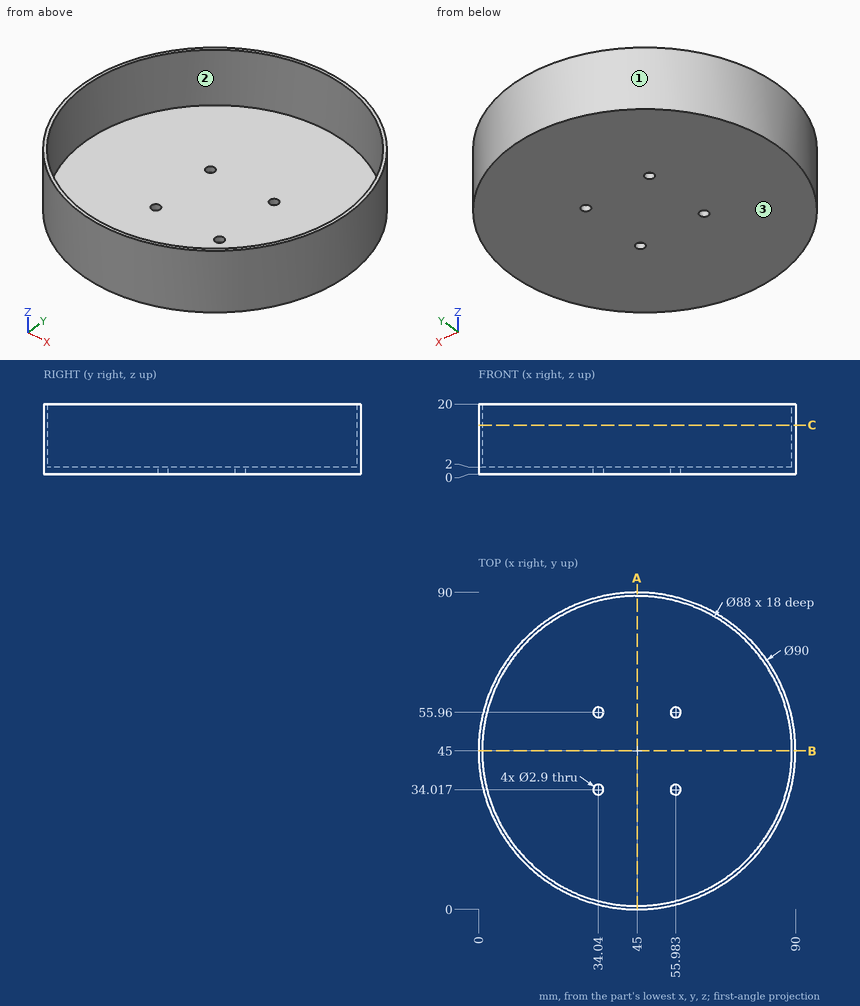
Study the drawing (mm; zero at the part's minimum x, y, z) and answer. Coordinates: 2 decimals unless noted, no trailing zeros. Order: outer loops, then holes, each group sorted by start corner. A loop starts at its lowest first (then second) coordinate and runs counter-clockwise, first axis right, second up. Notation, with made-up numbers: M 57,70.5 L 79,70.5 A22 cw 79,84.5 Z; hole C -12.75,-15 d8. An arc over 180 degrees is marked long. Answer as a JSON object with one key per item and string values. Group by question number.
1. Section C-C on z = 14 is taken. Write down the section's boundary in (x, y).
2. Flat-ended cylindrical pins translate along their axes: P1, Ø5, axis at x = 51, z = 17.5, coming from the +Y side; P2, Ø4, axis at x = 34.04, y = 55.96, coming from the +Z side; P3, Ø1.5, axis at x = 70, z = 9.5, coming from the +Y side. Find the tip coordinate at first contact, or state that the pin passes through.
3. Section A-A on x = 45 is taken. Write down the section's boundary in (y, z), then the cut area to 3 significant figures.
4. Determine the mould class of the marked faces 1, 2 and 3 for opening direction X: released by +X, released by -X, zero draft, split by the parting line, or undercut.
5. Straight lines are drawn through the part: line 1 (X direction, y = 44.5, z = 2.5); line 2 (Y direction, x = 44, z = 13); line 3 (X direction, y = 80.5, z = 10.5) (1 decimal). For each, find the intervals that lie inside material, in ascending order.
Values follow:
{
 "1": {"outline": "C 45,45 d90; hole C 45,45 d88"},
 "2": {"P1": "y = 89.86", "P2": "z = 2", "P3": "y = 82.91"},
 "3": {"outline": "M 0,0 L 90,0 L 90,20 L 89,20 L 89,2 L 1,2 L 1,20 L 0,20 Z", "area": "216 mm2"},
 "4": {"face 1": "split by the parting line", "face 2": "undercut", "face 3": "zero draft"},
 "5": {"line 1": "0 to 1, 89 to 90", "line 2": "0.01 to 1.01, 88.99 to 89.99", "line 3": "17.3 to 19, 71 to 72.7"}
}
